from build123d import *

# Parameters (mm, degrees)
BOSS_EXTRUDE1_DEPTH     = 127
CUT_EXTRUDE1_START      = -31.75
CUT_EXTRUDE1_DEPTH      = 28.575
CUT_EXTRUDE2_START      = 31.75
CUT_EXTRUDE2_DEPTH      = 28.575
SKETCH3_W               = 25.4
SKETCH3_H               = 50.8
CUT_EXTRUDE4_DEPTH      = 28.575
CUT_EXTRUDE7_DEPTH      = 140.18702407
CUT_EXTRUDE7_DEPTH_BACK = 140.18702407
CUT_EXTRUDE6_DEPTH      = 133.668601113
CUT_EXTRUDE6_DEPTH_BACK = 133.668601113
SKETCH5_R               = 1.5875
CUT_EXTRUDE9_DEPTH      = 133.824762172
CUT_EXTRUDE9_DEPTH_BACK = 133.824762172
SKETCH8_R               = 2.25
SKETCH9_W               = 25.4
SKETCH9_H               = 15.875
SKETCH9_R               = 1.5875
BOSS_EXTRUDE2_DEPTH     = 3.175
FILLET1_R               = 1.27


with BuildPart() as part:
    # Sketch1 → Boss-Extrude1 (new body)
    with BuildSketch(Plane(origin=(0, 0, 0), x_dir=(1, 0, 0), z_dir=(0, 1, 0))):
        Polygon((0, 0), (-25.4, 0), (-25.4, 6.985), (0, 50.979090512), align=None)
    extrude(amount=BOSS_EXTRUDE1_DEPTH)

    # Sketch2 → Cut-Extrude1 (cut)
    with BuildSketch(Plane(origin=(0, 63.5, 0), x_dir=(-1, 0, 0), z_dir=(0, -1, 0)).offset(CUT_EXTRUDE1_START)):
        Polygon((25.4, 6.985), (3.175, 45.479829198), (3.175, 3.175), (25.4, 3.175), align=None)
    extrude(amount=-CUT_EXTRUDE1_DEPTH, mode=Mode.SUBTRACT)

    # Sketch2<2> → Cut-Extrude2 (cut)
    with BuildSketch(Plane(origin=(0, 63.5, 0), x_dir=(-1, 0, 0), z_dir=(0, -1, 0)).offset(CUT_EXTRUDE2_START)):
        Polygon((25.4, 6.985), (3.175, 45.479829198), (3.175, 3.175), (25.4, 3.175), align=None)
    extrude(amount=CUT_EXTRUDE2_DEPTH, mode=Mode.SUBTRACT)

    # Sketch3 → Cut-Extrude4 (cut, symmetric)
    with BuildSketch(Plane(origin=(0, 63.5, 0), x_dir=(-1, 0, 0), z_dir=(0, -1, 0))):
        with Locations((12.7, 28.575)):
            Rectangle(SKETCH3_W, SKETCH3_H)
    extrude(amount=CUT_EXTRUDE4_DEPTH, both=True, mode=Mode.SUBTRACT)

    # Sketch6 → Cut-Extrude7 (cut, two sides: drawn at the far end of the back side and taken through both)
    with BuildSketch(Plane.XZ.offset(-CUT_EXTRUDE7_DEPTH_BACK)):
        Polygon((0, -31.929090512), (0, -50.979090512), (-10.998522628, -31.929090512), align=None)
    extrude(amount=CUT_EXTRUDE7_DEPTH + CUT_EXTRUDE7_DEPTH_BACK, mode=Mode.SUBTRACT)

    # Sketch5 → Cut-Extrude6 (cut, two sides: drawn at the far end of the back side and taken through both)
    with BuildSketch(Plane(origin=(0, 0, -3.175), x_dir=(-1, 0, 0), z_dir=(0, 0, -1)).offset(-CUT_EXTRUDE6_DEPTH_BACK)):
        with Locations((6.35, 84.1375)):
            Circle(SKETCH5_R)
        with Locations((19.05, 42.8625)):
            Circle(SKETCH5_R)
    extrude(amount=CUT_EXTRUDE6_DEPTH + CUT_EXTRUDE6_DEPTH_BACK, mode=Mode.SUBTRACT)

    # Sketch8 → Cut-Extrude9 (cut, two sides: drawn at the far end of the back side and taken through both)
    with BuildSketch(Plane.ZY.offset(3.175).offset(-CUT_EXTRUDE9_DEPTH_BACK)):
        with Locations((-19.229090512, 11)):
            Circle(SKETCH8_R)
        with Locations((-19.229090512, 116)):
            Circle(SKETCH8_R)
    extrude(amount=CUT_EXTRUDE9_DEPTH + CUT_EXTRUDE9_DEPTH_BACK, mode=Mode.SUBTRACT)

    # Sketch9 → Boss-Extrude2 (add)
    # profile 1 of 2: a face of its own
    with BuildSketch(Plane.XY):
        with Locations((-12.7, -7.9375)):
            Rectangle(SKETCH9_W, SKETCH9_H)
        with Locations((-12.7, -7.9375)):
            Circle(SKETCH9_R, mode=Mode.SUBTRACT)
    # profile 2 of 2: a face of its own
    with BuildSketch(Plane.XY):
        with Locations((-12.7, 134.9375)):
            Rectangle(SKETCH9_W, SKETCH9_H)
        with Locations(Location((-12.7, 134.9375, 0), (0, 0, 180))):
            Circle(SKETCH9_R, mode=Mode.SUBTRACT)
    extrude(amount=-BOSS_EXTRUDE2_DEPTH)

    # Fillet1
    fillet1_edges = [part.edges().sort_by_distance(p)[0] for p in [
        (0, 0, -17.552045256),
        (0, -15.875, -1.5875),
        (-25.4, -15.875, -1.5875),
        (-25.4, 127, -5.08),
        (0, 127, -17.552045256),
        (-25.4, 142.875, -1.5875),
        (0, 142.875, -1.5875),
        (-3.175, 109.5375, -3.175),
        (-14.2875, 95.25, -3.175),
        (-14.2875, 123.825, -3.175),
        (-3.175, 123.825, -17.552045256),
        (-3.175, 17.4625, -3.175),
        (-14.2875, 31.75, -3.175),
        (-14.2875, 3.175, -3.175),
        (-25.4, 92.075, -5.08),
        (-25.4, 34.925, -5.08),
        (-18.199261314, 34.925, -19.457045256),
        (-18.199261314, 92.075, -19.457045256),
        (-25.4, 0, -5.08),
        (0, 34.925, -17.552045256),
        (-5.499261314, 34.925, -31.929090512),
        (0, 92.075, -17.552045256),
        (-3.175, 3.175, -17.552045256),
        (-3.175, 31.75, -17.552045256),
        (-3.175, 95.25, -17.552045256),
        (-18.199261314, 0, -19.457045256),
        (-18.199261314, 127, -19.457045256),
        (-5.499261314, 0, -31.929090512),
        (-5.499261314, 127, -31.929090512),
        (-5.499261314, 92.075, -31.929090512),
        (0, 17.4625, -31.929090512),
        (0, 109.5375, -31.929090512),
    ]]
    fillet(fillet1_edges, radius=FILLET1_R)


solid = part.part
Model file for the job. Use its own axes, mm. A direction names the side the tool comes from. Give positions to 0.01 mm unless a question says otherwise; leave off trailing zeros. Write each loop counter-clockwise with the first axis right and the second up, starting at its lowest first coordinate (ties: lowest second). Pieces come first, ordered by that corner, then holes. Notation, with made-up numbers: (-4, -38) -> (37, -38) arc R24 cw to (37, -27) -> close; hole circle Ø8 at (12, 23). An arc over 180 degrees is marked (long way). Write item = value, one per line.
(1) Slice it at A-A, the plane y = 11. Give the cut face in (x, z) (3 decimals), then the cut area to 3 significant figures.
Determined:
outline = (-25.4, -3.175) -> (-4.445, -3.175) arc R1.27 cw to (-3.175, -4.445) -> (-3.175, -16.979) -> (0, -16.979) -> (0, 0) -> (-25.4, 0) -> close; (-3.175, -31.929) -> (-1.27, -31.929) arc R1.27 ccw to (0, -30.659) -> (0, -21.479) -> (-3.175, -21.479) -> close
area = 158 mm2
(2) Slice it at B-B, the plane y = 111. Give the cut face in (x, z) (3 decimals), then the cut area to 3 significant figures.
Determined:
outline = (-25.4, -3.175) -> (-4.445, -3.175) arc R1.27 cw to (-3.175, -4.445) -> (-3.175, -31.929) -> (-1.27, -31.929) arc R1.27 ccw to (0, -30.659) -> (0, 0) -> (-25.4, 0) -> close
area = 172 mm2
(3) Slice it at D-D, the plane y = 81. Give the cut face in (x, z) (3 decimals), then the cut area to 3 significant figures.
Determined:
outline = (-25.4, -3.175) -> (0, -3.175) -> (0, 0) -> (-25.4, 0) -> close
area = 80.6 mm2
(4) Mould opens along X. For faces 1 (the face through (-6.006, 82.588, -1.565)), 2 (the face through (-12, 123.825, -15)), 3 (the face through (-18.3, 124.76, -19.28)) say: released by +X, released by -X, zero draft, split by the parting line, or undercut.
Determined:
face_1 = undercut
face_2 = zero draft
face_3 = released by -X
(5) Flat gauge pins, fed straight in: P1, Ø13, axis at y = 108.5, z = -16, coming from the -X side (3 decimals); P2, Ø6.5, axis at x = -17.5, y = 111, coming from the -Z side (3 decimals); P3, Ø11.5, axis at x = -12, z = -11, coming from the +Y side; P4, Ø3, axis at x = -17, z = -27.5, coming from the +Y side. Where does each tip first touch, or does it go through?
Determined:
P1 = -3.175
P2 = -3.175
P3 = 127
P4 = through
(6) Tool access for faces 4 (the face through (-10, 127, -14)), 5 (the face through (-17.99, 92.46, -19.1)), 6 (the face through (-10, 92.075, -14)): list every direction of +Z, -Z, +X, -X, +Y, -Y with a clear straight run to the whole face (end or side of a thin tool).
Determined:
face_4 = -Z, +X, -X, +Y
face_5 = -Z, -X
face_6 = -Z, +X, -X
(7) Slice it at C-C, the plane x = -12.75. Give the number of separate pieces and of enclosed holes in the cut face, then the cut area to 3 significant figures.
Determined:
separate_pieces = 3
enclosed_holes = 0
area = 809 mm2
(8) Probe line 1 along Y through (x, z) = (-7.75, -23.5) (3 decimals); line 2 along Y through (x, z) = (-12.7, -1.95) (3 decimals); line 3 along Y through (x, z) = (-6.35, -0.65) (3 decimals). List the from-to ranges inside material, lowest first.
Determined:
line_1 = 0 to 3.175, 31.75 to 34.925, 92.075 to 95.25, 123.825 to 127
line_2 = -15.875 to -9.525, -6.35 to 133.35, 136.525 to 142.875
line_3 = -15.875 to 82.55, 85.725 to 142.875
